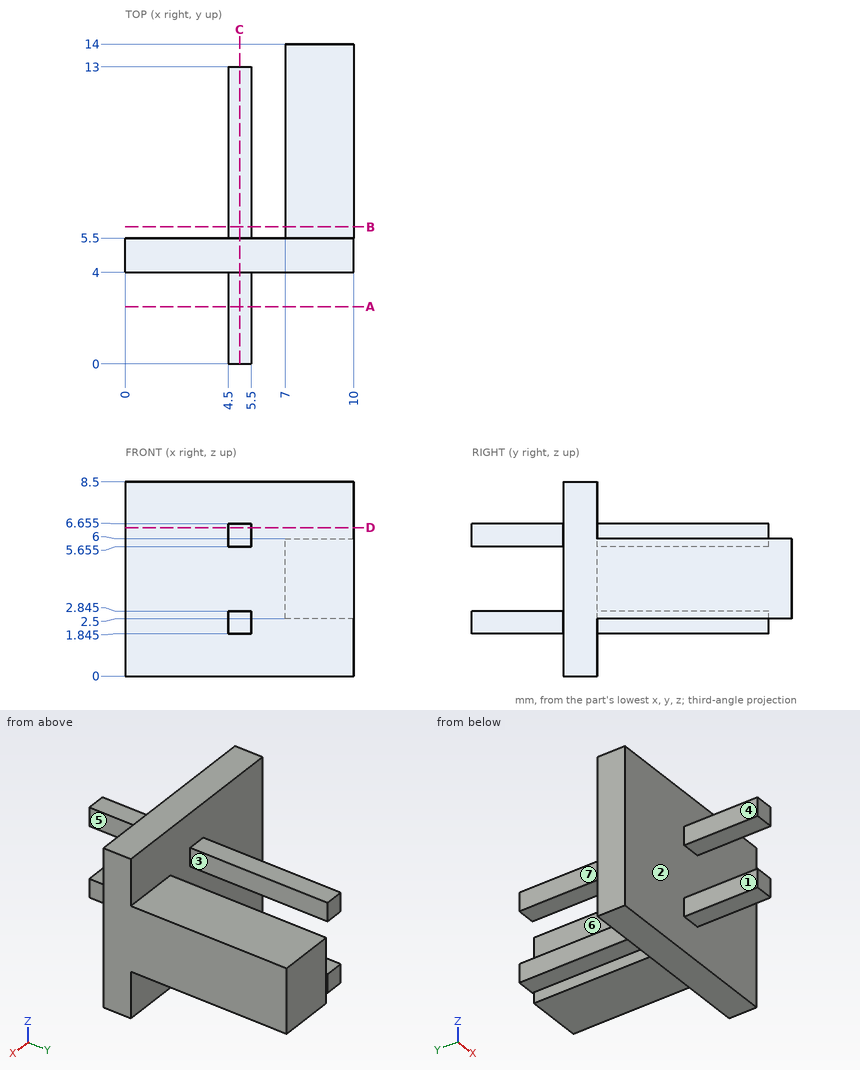
Drawing for the job (mm, zero at the part's lowest x, y, z). A direction names the side the tool comes from. Round coordinates to 2 decimals unless told otherwise and drop trailing zeros. Write each loop counter-clockwise with the first axis right and the second up, starting at its lowest first coordinate (ties: lowest second). Pieces come first, ordered by that corner, then holes. Notation, with made-up numbers: (51, 21) - (98, 21) arc R10 cw to (98, 38) - close; hole circle Ø2 at (-31.75, -12). An arc over 180 degrees is marked (long way). Write item = value, one per line. Start each with the question number.
Q1. Band-saw the part on D-D (z = 6.5). Give the cut face in (x, y).
Q2. Probe L1, parallel to X at y = 5.75, z = 5.75; L2, parallel to Y at x = 7.75, z = 7.5; L3, parallel to X at y = 3, z = 2.5. List the from-to ranges inside material, lowest first. Write a range as from..to.
Q3. Band-saw the part on C-C (x = 5). Give the cut face in (y, z) (3 decimals).
Q4. Which spindle directions (+Z, -Z, +X, -X, +Y, -Y) get a long thin tool onto all of the face, cutting with end or side? Do the marked faces 4, 5, 6 and 7. Say none if no direction does.
Q5. Band-saw the part on A-A (y = 2.5). Give the cut face in (x, z) (3 decimals).
Q6. Drop flat-ended pins along their axis: pin 1 (0.5 mm diameter, centred on x = 5, z = 2.5, fed in from +Y); pin 2 (0.5 mm diameter, centred on x = 5, y = 8.5, fed in from +Z) (3 decimals); pin 3 (0.8 mm diameter, centred on y = 9.5, z = 6, fed in from -X); pin 4 (1.1 mm diameter, centred on y = 11, z = 6.5, fed in from +X). Give the stop position or say it passes through.
Q7. Band-saw the part on B-B (y = 6). Give the cut face in (x, z) (3 decimals), then the cut area to 3 significant figures.
Q8. Mould opens along X. For the marked faces 1, 2 and 3 say: pulls with the +X half, pulls with the -X half, needs draft (parallel to the pull), parting line crosses it, or undercut.
Answers below:
q1.outline = (0, 4) - (4.5, 4) - (4.5, 0) - (5.5, 0) - (5.5, 4) - (10, 4) - (10, 5.5) - (5.5, 5.5) - (5.5, 13) - (4.5, 13) - (4.5, 5.5) - (0, 5.5) - close
q2.L1 = 4.5..5.5, 7..10
q2.L2 = 4..5.5
q2.L3 = 4.5..5.5
q3.outline = (0, 1.845) - (4, 1.845) - (4, 0) - (5.5, 0) - (5.5, 1.845) - (13, 1.845) - (13, 2.845) - (5.5, 2.845) - (5.5, 5.655) - (13, 5.655) - (13, 6.655) - (5.5, 6.655) - (5.5, 8.5) - (4, 8.5) - (4, 6.655) - (0, 6.655) - (0, 5.655) - (4, 5.655) - (4, 2.845) - (0, 2.845) - close
q4.face_4 = +Z, -Z, -X, -Y
q4.face_5 = +Z, -Z, +X, -Y
q4.face_6 = +Z, -Z, +Y
q4.face_7 = +Z, -Z, -X, +Y
q5.outline = (4.5, 1.845) - (5.5, 1.845) - (5.5, 2.845) - (4.5, 2.845) - close; (4.5, 5.655) - (5.5, 5.655) - (5.5, 6.655) - (4.5, 6.655) - close
q6.pin_1 = 13
q6.pin_2 = 6.655
q6.pin_3 = 4.5
q6.pin_4 = 10
q7.outline = (4.5, 1.845) - (5.5, 1.845) - (5.5, 2.845) - (4.5, 2.845) - close; (4.5, 5.655) - (5.5, 5.655) - (5.5, 6.655) - (4.5, 6.655) - close; (7, 2.5) - (10, 2.5) - (10, 6) - (7, 6) - close
q7.area = 12.5 mm2
q8.face_1 = pulls with the -X half
q8.face_2 = needs draft
q8.face_3 = undercut
